The listing builds one solid part. Answer for the finished solid, in the listing's coordinates (mm). A direction names the side the tool comes from. Round coordinates to 2 decimals unless told otherwise and drop trailing zeros. Loops run counter-clockwise (first coordinate to the right, second up) from the corner with the lowest first, then second, coordinate; pieces in that order, holes last. Notation, with made-up numbers: (-33.75, -28) -> (0.25, -28) arc R19 ccw to (0.25, -10) -> close; hole circle Ø10 at (80, -6). An arc over 180 degrees is marked (long way). Answer in a Markdown table with one row per item. Add a question column.
```python
from build123d import *

# Parameters (mm, degrees)
SKETCH1_R           = 3
BOSS_EXTRUDE1_DEPTH = 2
SKETCH2_R           = 1.5
BOSS_EXTRUDE2_DEPTH = 10
SKETCH3_W           = 0.9
SKETCH3_H           = 0.9
SKETCH3_W_2         = 1.05
SKETCH3_H_2         = 1.05
CUT_EXTRUDE1_DEPTH  = 1.9
FILLET1_R           = 0.4


with BuildPart() as part:
    # Sketch1 → Boss-Extrude1 (new body)
    with BuildSketch(Plane(origin=(0, 0, 0), x_dir=(1, 0, 0), z_dir=(0, 1, 0))):
        Circle(SKETCH1_R)
    extrude(amount=BOSS_EXTRUDE1_DEPTH)

    # Sketch2 → Boss-Extrude2 (add)
    with BuildSketch(Plane(origin=(0, 2, 0), x_dir=(1, 0, 0), z_dir=(0, 1, 0))):
        Circle(SKETCH2_R)
    extrude(amount=BOSS_EXTRUDE2_DEPTH)

    # Sketch3 → Cut-Extrude1 (cut)
    with BuildSketch(Plane(origin=(0, 0, 0), x_dir=(-1, 0, 0), z_dir=(0, -1, 0))):
        Rectangle(SKETCH3_W, SKETCH3_H)
        with Locations((0.975, 0)):
            Rectangle(SKETCH3_W_2, SKETCH3_H)
        with Locations((0, -0.975)):
            Rectangle(SKETCH3_W, SKETCH3_H_2)
        with Locations((-0.975, 0)):
            Rectangle(SKETCH3_W_2, SKETCH3_H)
        with Locations((0, 0.975)):
            Rectangle(SKETCH3_W, SKETCH3_H_2)
    extrude(amount=-CUT_EXTRUDE1_DEPTH, mode=Mode.SUBTRACT)

    # Fillet1
    fillet1_edges = [part.edges().sort_by_distance(p)[0] for p in [
        (-3, 0, 0),
        (-3, 2, 0),
    ]]
    fillet(fillet1_edges, radius=FILLET1_R)


solid = part.part
```
Item 1: Flat-ended cylindrical pins translate along their axes: P1, Ø1.2, axis at y = 1, z = -1, coming from the +X side; P2, Ø0.5, axis at x = -1, y = 1, coming from the -Z side; P3, Ø0.5, axis at y = 1, z = -1, coming from the -X side. Find the tip coordinate at first contact, or state that the pin passes through.
Item 2: For faces 1 (the flat face through (1, 1, -0.45)), 2 (the flat face through (2, 2, 0)), 3 (the flat face through (1, 0, 1)), determine the directions among +Z, -Z, +X, -X, +Y, -Y from which every point of the face is accessible in a straight line to the end or side of a thin tool.
Item 3: Section B-B, the plane z = 0 is taken. Write down the section's boundary in (x, y).
Item 4: The mould has two halves that part along Z. Classify faces 4 (the flat face through (1.5, 1, 0)), 5 (the cylindrical face through (-1.5, 6.93, -0.07)), 6 (the flat face through (0, 12, 0)): +Z half, -Z half, draft (parallel to the pull), parting line (faces both ways), or undercut.
Item 5: Section C-C, the plane y = 8 is taken. Write down the section's boundary in (x, z), and give its area (3 significant figures).
Item 6: Consider L1, parallel to Y at x = -0.35, z = -0.1; L2, parallel to Y at x = 1.15, z = 1.6; L3, parallel to Z at x = 0.15, y = 1. Determine where each line is inside the solid, lowest interval first. Write a range as from..to.
Item 7: Section A-A, the plane x = 0 is taken. Write down the section's boundary in (y, z), and give its area (3 significant figures).
Here are the results:
| question | item | result |
|---|---|---|
| 1 | P1 | stops at x = 2.97 |
| 1 | P2 | stops at z = -2.9 |
| 1 | P3 | stops at x = -2.9 |
| 2 | face 1 | -Y |
| 2 | face 2 | +Y |
| 2 | face 3 | +Z, -Z, +X, -X, -Y |
| 3 | outline | (-3, 0.4) arc R0.4 ccw to (-2.6, 0) -> (-1.5, 0) -> (-1.5, 1.9) -> (1.5, 1.9) -> (1.5, 0) -> (2.6, 0) arc R0.4 ccw to (3, 0.4) -> (3, 1.6) arc R0.4 ccw to (2.6, 2) -> (1.5, 2) -> (1.5, 12) -> (-1.5, 12) -> (-1.5, 2) -> (-2.6, 2) arc R0.4 ccw to (-3, 1.6) -> close |
| 4 | face 4 | undercut |
| 4 | face 5 | parting line |
| 4 | face 6 | draft |
| 5 | outline | circle Ø3 at (0, 0) |
| 5 | area | 7.07 mm² |
| 6 | L1 | y = 1.9..12 |
| 6 | L2 | y = 0..2 |
| 6 | L3 | z = -3..-1.5, 1.5..3 |
| 7 | outline | (0, -2.6) arc R0.4 ccw to (0.4, -3) -> (1.6, -3) arc R0.4 ccw to (2, -2.6) -> (2, -1.5) -> (12, -1.5) -> (12, 1.5) -> (2, 1.5) -> (2, 2.6) arc R0.4 ccw to (1.6, 3) -> (0.4, 3) arc R0.4 ccw to (0, 2.6) -> (0, 1.5) -> (1.9, 1.5) -> (1.9, -1.5) -> (0, -1.5) -> close |
| 7 | area | 36.2 mm² |
